Could you check a few things on this model? Use its own coordinates, in mm. A direction names the side the tool comes from. Give positions to 0.01 mm unless a question says otherwise; leave off trailing zeros. Order: outer loops, then holes, each group sorted by start corner. A loop starts at its lowest first (then second) coordinate and runs counter-clockwise, first axis right, second up. Notation, with made-up numbers: M 82.5,84.5 L 133.5,84.5 A32 cw 133.5,112.5 Z; hole C 0.25,-33 d6. An arc over 180 degrees is marked long. Use a Markdown table: item, result. Add a question column.
Item 1: Suppose I cut it at B-B on z = 0. Write out the boundary of the cut face in (x, y).
Item 2: Suppose I cut it at A-A on x = 0. Write out the boundary of the cut face in (y, z), plus the area to 3 significant figures.
Item 3: I'm going to push flat-ended pins straight in: pin 1 Ø3 at (x, y) = (-9.5, 8.5) entering from +Z; pin 2 Ø3 at (x, y) = (-17, 3) entering from +Z; pin 3 Ø1.3 at (x, y) = (16.5, 5) entering from +Z. Where does each tip first touch, or does it pass through?
Item 4: If we mould it in two halves opening along X, with no side actions, what happens to faces 1 (the face through (5, 10, 4)), 2 (the face through (20, 5, 0)), 3 (the face through (-15, 5, 0))? For each: released by +X, released by -X, zero draft, split by the parting line, or undercut.
Item 5: If I drill on L1, parallel to X at y = 4.5, z = 0; L2, parallel to X at y = 5.25, z = 2; L3, parallel to Z at x = 1, y = 3.5, over which ranges is the centre line in solid material (lowest first)? Write a range as from..to.
Item 6: Suppose I cut it at D-D on x = -16. Write out the boundary of the cut face in (y, z), plus the area to 3 significant figures.
Item 7: Suppose I cut it at C-C on y = 8.75. Write out the boundary of the cut face in (x, z), plus the area to 3 significant figures.
Item 8: For faces 4 (the face through (-17.6, 5, 0)), 5 (the face through (-20, 5, 0)), which set-ups out of +Z, -Z, +X, -X, +Y, -Y let a thin tool reach every point of the face, with its end or its side?
from build123d import *

# Parameters (mm, degrees)
SKETCH1_W           = 40
SKETCH1_H           = 20
SKETCH1_R           = 5
SKETCH1_W_2         = 2.6
SKETCH1_H_2         = 10
BOSS_EXTRUDE1_DEPTH = 10


with BuildPart() as part:
    # Sketch1 → Boss-Extrude1 (new body)
    # profile 1 of 2: a face of its own
    with BuildSketch(Plane(origin=(0, 0, 0), x_dir=(1, 0, 0), z_dir=(0, 1, 0))):
        Rectangle(SKETCH1_W, SKETCH1_H)
        with Locations(Location((0, 0, 0), (0, 0, 270))):
            Circle(SKETCH1_R, mode=Mode.SUBTRACT)
        with Locations((16.3, 0)):
            Rectangle(SKETCH1_W_2, SKETCH1_H_2, mode=Mode.SUBTRACT)
        with Locations((-16.3, 0)):
            Rectangle(SKETCH1_W_2, SKETCH1_H_2, mode=Mode.SUBTRACT)
    # profile 2 of 2: a face of its own
    with BuildSketch(Plane(origin=(0, 0, 0), x_dir=(1, 0, 0), z_dir=(0, 1, 0))):
        with BuildLine():
            Line((-20, -10), (20, -10))
            ThreePointArc((20, -10), (0, -18.284271247), (-20, -10))
        make_face()
    extrude(amount=BOSS_EXTRUDE1_DEPTH)


solid = part.part
Findings below:
| question | item | result |
|---|---|---|
| 1 | outline | M -20,0 L -17.6,0 L -17.6,10 L -20,10 Z; M -15,0 L -5,0 L -5,10 L -15,10 Z; M 5,0 L 15,0 L 15,10 L 5,10 Z; M 17.6,0 L 20,0 L 20,10 L 17.6,10 Z |
| 2 | outline | M 0,-10 L 10,-10 L 10,-5 L 0,-5 Z; M 0,5 L 10,5 L 10,18.28 L 0,18.28 Z |
| 2 | area | 183 mm^2 |
| 3 | pin 1 | stops at z = 17.13 |
| 3 | pin 2 | stops at z = 13.66 |
| 3 | pin 3 | stops at z = 13.43 |
| 4 | face 1 | zero draft |
| 4 | face 2 | released by +X |
| 4 | face 3 | undercut |
| 5 | L1 | x = -20..-17.6, -15..-5, 5..15, 17.6..20 |
| 5 | L2 | x = -20..-17.6, -15..-4.58, 4.58..15, 17.6..20 |
| 5 | L3 | z = -10..-4.9, 4.9..18.27 |
| 6 | outline | M 0,-10 L 10,-10 L 10,-5 L 0,-5 Z; M 0,5 L 10,5 L 10,13.32 L 0,13.32 Z |
| 6 | area | 133 mm^2 |
| 7 | outline | M -20,-10 L 20,-10 L 20,10 A28.28 ccw -20,10 Z; hole M -17.6,-5 L -15,-5 L -15,5 L -17.6,5 Z; hole C 0,0 d10; hole M 15,-5 L 17.6,-5 L 17.6,5 L 15,5 Z |
| 7 | area | 898 mm^2 |
| 8 | face 4 | +Y, -Y |
| 8 | face 5 | +Z, -Z, -X, +Y, -Y |
